Geometry check sheet. Reference: the model listing, model coordinates, mm. Face numbers are marked on the shaded views. A direction names the side the tool comes from. Coordinates: 2 decimals unless noted, no trailing zeros. Loops run counter-clockwise (first coordinate to the right, second up) from the corner with the lowest first, then second, coordinate; pieces in that order, holes last. Notation, with made-up numbers: (-25.5, 76) - (-6.5, 76) arc R21 cw to (-6.5, 91) - close; hole circle Ø9 at (50, -29.5). An arc over 180 degrees is marked (long way). Write each question's results on one line, items separated by ' | '. Start each with the question number.
(1) Material ranges on probe 1 along Z at (x, y) = (-3.25, -5); probe 2 along Z at (x, y) = (1, -4.25); probe 3 along Z at (x, y) = (-1.5, 6.5), recorded low to high.
(2) Access from +Z, -Z, +X, -X, +Y, -Y to the whole of each face (thin tool, end or side, straight path). Record for the marked faces 1, 2 and 3.
(3) Sectioned sample at C-C (z = 8). Enter the section's corners in (x, y).
(4) Go/stop test with flat-tipped pins: pin 1 Ø3 at (x, y) = (-4.5, -0.5) entering from +Z; pin 2 Ø1.5 at (x, z) = (-0.5, 22.5) entering from -Y; pin 3 Ø2 at (y, z) = (-5, 12.5) entering from -X. Record where each tip stops, or that it passes through.
(5) Sectioned sample at A-A (x = -5.5). State how many separate pieces and enclosed holes the cut face has, plus the area to 3 significant figures.
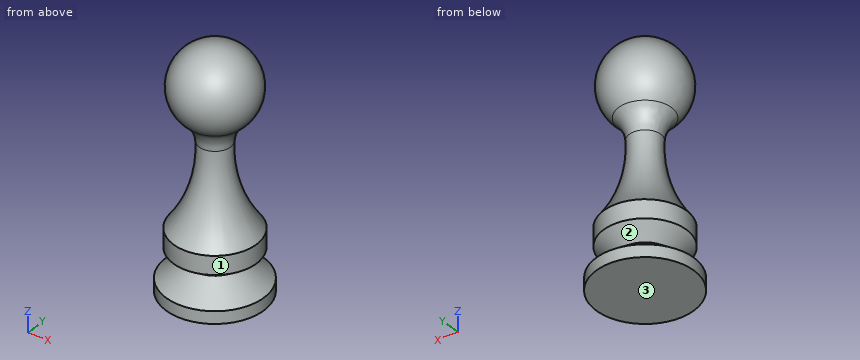
from build123d import *

# Parameters (mm, degrees)
F2_R = 5


with BuildPart() as f1:
    # F0 (on Front) → F1 (revolve)
    with BuildSketch(Plane.XZ):
        with BuildLine():
            Line((-8, 0), (0, 0))
            Line((0, 0), (0, 9.87))
            Line((0, 9.87), (0, 26.07))
            Line((0, 26.07), (0, 32))
            Line((0, 32), (0, 38.59))
            ThreePointArc((0, 38.59), (-6.422881, 33.474686), (-2.874578, 26.07))
            ThreePointArc((-2.874578, 26.07), (-3.123928, 17.559362), (-6.78, 9.87))
            Line((-6.78, 9.87), (-6.78, 6.87))
            Line((-6.78, 6.87), (-4, 4.935))
            Line((-4, 4.935), (-8, 2))
            Line((-8, 2), (-8, 0))
        make_face()
    revolve(axis=Axis((0, 0, 35.295), (0, 0, 1)))

    # F2
    f2_edges = [f1.edges().sort_by_distance(p)[0] for p in [
        (2.874578, 0, 26.07),
        (-6.422881, 0, 33.474686),
    ]]
    fillet(f2_edges, radius=F2_R)


solid = f1.part
Outcome:
1) probe 1: z = 0 to 3.49, 6.3 to 11.02, 29.2 to 34.8 | probe 2: z = 0 to 4.67, 5.19 to 13.93, 27.06 to 36.94 | probe 3: z = 0 to 2.98, 6.79 to 10.01
2) face 1: +Z | face 2: none | face 3: -Z, +X, -X, +Y, -Y
3) outline: circle Ø13.56 at (0, 0)
4) pin 1: stops at z = 37.85 | pin 2: stops at y = -2.56 | pin 3: stops at x = -3.42
5) separate pieces: 3 | enclosed holes: 0 | area: 116 mm2
